from build123d import *

# Parameters (mm, degrees)
BOSS_EXTRUDE1_DEPTH = 33.02
SHELL1_T            = -2.54
CUT_EXTRUDE1_REACH  = 570.92
SKETCH2_W           = 27.94
SKETCH2_H           = 27.94
SKETCH3_R           = 6.35
CUT_EXTRUDE2_DEPTH  = 540.640918389
SKETCH4_R           = 6.35
CUT_EXTRUDE3_DEPTH  = 540.640918389


with BuildPart() as part:
    # Sketch1 → Boss-Extrude1 (new body)
    with BuildSketch(Plane.XY):
        with BuildLine():
            Line((0, 0), (0, -33.02))
            Line((0, -33.02), (215.9, -33.02))
            ThreePointArc((215.9, -33.02), (242.840768363, -21.860768363), (254, 5.08))
            Line((254, 5.08), (254, 474.98))
            Line((254, 474.98), (220.98, 474.98))
            Line((220.98, 474.98), (220.98, 38.1))
            ThreePointArc((220.98, 38.1), (209.820768363, 11.159231637), (182.88, 0))
            Line((182.88, 0), (0, 0))
        make_face()
    extrude(amount=BOSS_EXTRUDE1_DEPTH)

    # Shell1
    shell1_openings = [part.faces().sort_by_distance(p)[0] for p in [
        (0, -16.51, 16.51),
    ]]
    offset(amount=SHELL1_T, openings=shell1_openings, kind=Kind.INTERSECTION)

    # Sketch2 → Cut-Extrude1 (cut, up to next)
    with BuildSketch(Plane(origin=(0, 474.98, 0), x_dir=(1, 0, 0), z_dir=(0, 1, 0)), mode=Mode.PRIVATE) as cut_extrude1_sk1:
        with Locations((237.49, -16.51)):
            Rectangle(SKETCH2_W, SKETCH2_H)
    cut_extrude1_tool1 = extrude(cut_extrude1_sk1.sketch, amount=-CUT_EXTRUDE1_REACH, mode=Mode.PRIVATE) & part.part
    add(cut_extrude1_tool1.solids().sort_by_distance((237.49, 474.98, 16.51))[0], mode=Mode.SUBTRACT)

    # Sketch3 → Cut-Extrude2 (cut, through all)
    with BuildSketch(Plane.XY.offset(33.02)):
        with Locations((50.8, -16.51)):
            Circle(SKETCH3_R)
        with Locations((152.4, -16.51)):
            Circle(SKETCH3_R)
    extrude(amount=-CUT_EXTRUDE2_DEPTH, mode=Mode.SUBTRACT)

    # Sketch4 → Cut-Extrude3 (cut, through all)
    with BuildSketch(Plane.XY.offset(33.02)):
        with Locations((237.49, 449.58)):
            Circle(SKETCH4_R)
    extrude(amount=-CUT_EXTRUDE3_DEPTH, mode=Mode.SUBTRACT)


solid = part.part
Geometry check sheet. Reference: the model listing, model coordinates, mm. A direction names the side the tool comes from. Give positions to 0.01 mm unless a question says otherwise; leave off trailing zeros. Order: outer loops, then holes, each group sorted by start corner. A loop starts at its lowest first (then second) coordinate and runs counter-clockwise, first axis right, second up. Notation, with made-up numbers: M -26.5,9.25 L 14.5,9.25 A16 ccw 14.5,38.25 Z; hole C 10.5,8.5 d3. An arc over 180 degrees is marked long. Use a Markdown table: item, result.
Item 1: Tool access check on faces 1 (the flat face through (251.46, 237, 16)), 2 (the flat face through (93, 0, 16)), 3 (the flat face through (93, -2.54, 16)). Record the directions out of +Z, -Z, +X, -X, +Y, -Y that give a thin tool (end or side, any length) a straight path to the whole face; none if there is none.
Answers follow:
| item | result |
|---|---|
| face 1 | +Y |
| face 2 | +Z, -Z, -X, +Y |
| face 3 | -X |
Item 2: Section check A-A (z = 25.5). Record the cut outline in (x, y).
Answers follow:
| item | result |
|---|---|
| outline | M 0,-33.02 L 215.9,-33.02 A38.1 ccw 254,5.08 L 254,474.98 L 251.46,474.98 L 251.46,5.08 A35.56 cw 215.9,-30.48 L 0,-30.48 Z; M 0,-2.54 L 182.88,-2.54 A40.64 ccw 223.52,38.1 L 223.52,474.98 L 220.98,474.98 L 220.98,38.1 A38.1 cw 182.88,0 L 0,0 Z |
Item 3: Depth check by flat-ended pin: P1, Ø1.5, axis at y = 74, z = 11, coming from the -X side; P2, Ø7.5, axis at x = 237.49, y = 449.58, coming from the -Z side; P3, Ø8, axis at x = 210, z = 22.5, coming from the +Y side; P4, Ø14.5, axis at x = 50.8, y = -16.51, coming from the +Z side. Enter the tip coordinate at first touch or a pass-through.
Answers follow:
| item | result |
|---|---|
| P1 | stops at x = 220.98 |
| P2 | passes through |
| P3 | stops at y = 16.12 |
| P4 | stops at z = 33.02 |
Item 4: Material ranges on line 1 along X through (y, z) = (77.5, 23.5); line 2 along Y through (x, z) = (18, 23); line 3 along X through (y, z) = (-16, 31), recorded low to high.
Answers follow:
| item | result |
|---|---|
| line 1 | x = 220.98 to 223.52, 251.46 to 254 |
| line 2 | y = -33.02 to -30.48, -2.54 to 0 |
| line 3 | x = 0 to 44.47, 57.13 to 146.07, 158.73 to 247.64 |
Item 5: Section check D-D (x = 81). Record the cut outline in (y, z), and give its area (3 significant figures).
Answers follow:
| item | result |
|---|---|
| outline | M -33.02,0 L 0,0 L 0,33.02 L -33.02,33.02 Z; hole M -30.48,2.54 L -2.54,2.54 L -2.54,30.48 L -30.48,30.48 Z |
| area | 310 mm2 |
Item 6: Section check B-B (x = 152.4). Record the cut outline in (y, z), and give its area (3 significant figures).
Answers follow:
| item | result |
|---|---|
| outline | M -33.02,0 L -22.86,0 L -22.86,2.54 L -30.48,2.54 L -30.48,30.48 L -22.86,30.48 L -22.86,33.02 L -33.02,33.02 Z; M -10.16,0 L 0,0 L 0,33.02 L -10.16,33.02 L -10.16,30.48 L -2.54,30.48 L -2.54,2.54 L -10.16,2.54 Z |
| area | 245 mm2 |
Item 7: Draft check along Z on faces 4 (the cylindrical face through (211.93, 9.68, 16.31)), 5 (the flat face through (230, 147, 0)), 6 (the flat face through (106, -30.48, 16)), 7 (the cylindrical face through (236.663, 455.876, 1.288)). Enter one of: +Z half, -Z half, draft (parallel to the pull), parting line (faces both ways), or undercut.
Answers follow:
| item | result |
|---|---|
| face 4 | undercut |
| face 5 | -Z half |
| face 6 | undercut |
| face 7 | draft |
Item 8: Section check C-C (y = 427.5). Record the cut outline in (x, z), and give its area (3 significant figures).
Answers follow:
| item | result |
|---|---|
| outline | M 220.98,0 L 254,0 L 254,33.02 L 220.98,33.02 Z; hole M 223.52,2.54 L 251.46,2.54 L 251.46,30.48 L 223.52,30.48 Z |
| area | 310 mm2 |
